```python
from build123d import *

# Parameters (mm, degrees)
BOSS_EXTRUDE1_DEPTH = 1.25
SKETCH2_W           = 1
SKETCH2_H           = 0.325
BOSS_EXTRUDE2_DEPTH = 2
SKETCH3_W           = 1
SKETCH3_H           = 0.325
BOSS_EXTRUDE3_DEPTH = 2
BOSS_EXTRUDE7_DEPTH = 1
BOSS_EXTRUDE8_DEPTH = 1


with BuildPart() as part:
    # Sketch1 → Boss-Extrude1 (new body)
    with BuildSketch(Plane.XY):
        Polygon((1, 0), (9, 0), (9, -0.325), (10, -0.325), (10, -1), (17, -1), (17, 1), (10, 1), (0, 1), (-7, 1), (-7, -1), (0, -1), (0, -0.325), (1, -0.325), align=None)
    extrude(amount=BOSS_EXTRUDE1_DEPTH)

    # Sketch2 → Boss-Extrude2 (add)
    with BuildSketch(Plane.XY.offset(1.25)):
        with Locations((0.5, -0.1625)):
            Rectangle(SKETCH2_W, SKETCH2_H)
        with Locations((9.5, -0.1625)):
            Rectangle(SKETCH2_W, SKETCH2_H)
    extrude(amount=BOSS_EXTRUDE2_DEPTH)

    # Sketch3 → Boss-Extrude3 (add)
    with BuildSketch(Plane(origin=(0, 0, 0), x_dir=(-1, 0, 0), z_dir=(0, 0, -1))):
        with Locations((-9.5, -0.1625)):
            Rectangle(SKETCH3_W, SKETCH3_H)
        with Locations((-0.5, -0.1625)):
            Rectangle(SKETCH3_W, SKETCH3_H)
    extrude(amount=BOSS_EXTRUDE3_DEPTH)

    # Sketch7 → Boss-Extrude7 (add)
    with BuildSketch(Plane(origin=(10, 0, 0), x_dir=(0, 0, -1), z_dir=(1, 0, 0))):
        Polygon((-3.25, 0), (-1.25, 1), (-1.25, 0), (-1.25, -0.325), (-3.25, -0.325), align=None)
        Polygon((2, 0), (0, 1), (0, 0), align=None)
    extrude(amount=-BOSS_EXTRUDE7_DEPTH)

    # Sketch8 → Boss-Extrude8 (add)
    with BuildSketch(Plane.ZY):
        Polygon((-2, 0), (0, 1), (0, 0), align=None)
        Polygon((1.25, 1), (1.25, 0), (3.25, 0), align=None)
    extrude(amount=-BOSS_EXTRUDE8_DEPTH)


solid = part.part
```
Here's how the part is built. I have some questions about the finished solid (model axes, mm). A direction names the side the tool comes from. Give positions to 0.01 mm unless a question says otherwise; leave off trailing zeros. Order: outer loops, then holes, each group sorted by start corner. A loop starts at its lowest first (then second) coordinate and runs counter-clockwise, first axis right, second up. Notation, with made-up numbers: (51, 69.5) -> (100, 69.5) arc R16 cw to (100, 79.5) -> close; hole circle Ø10 at (-7, 16.5). An arc over 180 degrees is marked (long way). Use CSV: the item, a comma, the result in double quotes. Start each with the question number.
Item 1: Suppose I cut it at D-D (x = -1.25). List the corners of the cut face in (y, z) for me.
Item 2: On a 3-axis mill with a long thin cutter (end or side, diameter ignored), from which of +Z, -Z, +X, -X, +Y, -Y can I reach the whole of each face in a straight line? I mean faces 1 (the flat face through (0, 0, -1)), 2 (the flat face through (13, 0, 1.25)), 3 (the flat face through (9.5, -0.325, 0.7)). Say none if no direction works.
Item 3: Thinking about a two-plate mould opening in X: for faces 4 (the flat face through (-4, 0, 1.25)), 5 (the flat face through (4.9, 0.5, 0)), 6 (the flat face through (10, 0, -1)), 7 (the flat face through (0.5, -0.325, 0.7)), which applies, pulls with the +X half, pulls with the -X half, needs draft (parallel to the pull), parting line crosses it, or undercut?
Item 4: Suppose I cut it at C-C (y = 0.8). List the corners of the cut face in (x, z) for me.
Item 5: Suppose I cut it at B-B (y = -0.55). List the corners of the cut face in (x, z) for me, and give its area (3 significant figures).
Item 6: Suppose I cut it at A-A (z = -0.3). List the corners of the cut face in (x, y) for me (3 decimals), and give its area (3 significant figures).
Item 7: I'm going to push flat-ended pins straight in: P1, Ø0.7, axis at y = 0.5, z = -1.5, coming from the -X side; P2, Ø1.4, axis at x = 5.5, z = 0.5, coming from the -Y side; P3, Ø1.1, axis at x = 5, y = 0.5, coming from the -Z side. Where does each tip first touch, or does it pass through?
Item 8: If I drill on probe 1 along X at (y, z) = (0.55, -0.25); probe 2 along Z at (x, y) = (-5.25, 0.8); probe 3 along Z at (x, y) = (0.5, 0.65), over which ranges is the centre line in solid material (lowest first)? Write a range as [from, to].
Answer block:
1,outline,"(-1, 0) -> (1, 0) -> (1, 1.25) -> (-1, 1.25) -> close"
2,face 1,"-Z, -X, +Y, -Y"
2,face 2,"+Z, +X, +Y, -Y"
2,face 3,"+Z, -Z, -Y"
3,face 4,"needs draft"
3,face 5,"undercut"
3,face 6,"pulls with the +X half"
3,face 7,"undercut"
4,outline,"(-7, 0) -> (0, 0) -> (0, -0.4) -> (1, -0.4) -> (1, 0) -> (9, 0) -> (9, -0.4) -> (10, -0.4) -> (10, 0) -> (17, 0) -> (17, 1.25) -> (10, 1.25) -> (10, 1.65) -> (9, 1.65) -> (9, 1.25) -> (1, 1.25) -> (1, 1.65) -> (0, 1.65) -> (0, 1.25) -> (-7, 1.25) -> close"
5,outline,"(-7, 0) -> (0, 0) -> (0, 1.25) -> (-7, 1.25) -> close; (10, 0) -> (17, 0) -> (17, 1.25) -> (10, 1.25) -> close"
5,area,"17.5 mm^2"
6,outline,"(0, -0.325) -> (1, -0.325) -> (1, 0.85) -> (0, 0.85) -> close; (9, -0.325) -> (10, -0.325) -> (10, 0.85) -> (9, 0.85) -> close"
6,area,"2.35 mm^2"
7,P1,"stops at x = 0"
7,P2,"stops at y = 0"
7,P3,"stops at z = 0"
8,probe 1,"x = [0, 1], [9, 10]"
8,probe 2,"z = [0, 1.25]"
8,probe 3,"z = [-0.7, 1.95]"
